Could you check a few things on this model? Use its own coordinates, in mm. Give positions to 0.01 mm unless a question says otherwise; leave off trailing zeros. Loops run counter-clockwise (first coordinate to the right, second up) from the corner with the lowest first, then second, coordinate; pieces in that order, holes last. Notation, with made-up numbers: (27.5, -37.5) - (55.5, -37.5) arc R25 cw to (55.5, -3.5) - close; hole circle Ø1 at (60.5, -20.75). An arc over 180 degrees is marked (long way). Write each question's results on one line, items separated by ' | '. Start each with the question number.
(1) Suppose I cut it at B-B (y = 0.6). Count the separate pieces of the cut face and the enclosed holes in it, and give its area (3 significant figures).
(2) I need wall thicknesses on line 1 (X direction, y = 0.95, z = 8); line 2 (X direction, y = 0.8, z = 3.81); line 3 (X direction, y = 1, z = -2.54). Which ranges of each line are inside material? Lowest first, please.
(3) For pin 1 (5 mm diameter, centred on x = -8, z = 8, fed in from -Y); pin 2 (3 mm diameter, centred on x = 8, z = 8, fed in from +Y), each with a flat end and sliding along its axis, tell me the tip position at first contact or that it passes through.
(4) Suppose I cut it at D-D (z = 1.5). Please give me the cut outline in (x, y), and give its area (3 significant figures).
(5) If we mould it in two halves opening along Z, with no side actions, what happens to faces 1 (the face through (-8.97, 0.79, 6.73)), 2 (the face through (10.737, 0.789, 10.438)), 3 (the face through (11.65, 1, 0))? For each: released by +Z, released by -Z, zero draft, split by the parting line, or undercut.
(6) Suppose I cut it at C-C (x = -9). Please give me the cut outline in (y, z), and give its area (3 significant figures).
(7) Suppose I cut it at A-A (z = -3.81). Please give me the cut outline in (x, y).
from build123d import *

# Parameters (mm, degrees)
SKETCH_1_R      = 1.6
SKETCH_1_R_2    = 0.5
EXTRUDE_1_DEPTH = 1.6


with BuildPart() as part:
    # Эскиз1 → Бобышка-Вытянуть1 (new body)
    with BuildSketch(Plane(origin=(0, 0, 0), x_dir=(1, 0, 0), z_dir=(0, 1, 0))):
        with BuildLine():
            Line((-8.45, 11.4), (8.45, 11.4))
            ThreePointArc((8.45, 11.4), (10.7127417, 10.4627417), (11.65, 8.2))
            Line((11.65, 8.2), (11.65, -8.2))
            ThreePointArc((11.65, -8.2), (10.7127417, -10.4627417), (8.45, -11.4))
            Line((8.45, -11.4), (-8.45, -11.4))
            ThreePointArc((-8.45, -11.4), (-10.7127417, -10.4627417), (-11.65, -8.2))
            Line((-11.65, -8.2), (-11.65, 8.2))
            ThreePointArc((-11.65, 8.2), (-10.7127417, 10.4627417), (-8.45, 11.4))
        make_face()
        with Locations(Location((-8, 8, 0), (0, 0, 270))):
            Circle(SKETCH_1_R, mode=Mode.SUBTRACT)
        with Locations(Location((8, 8, 0), (0, 0, 270))):
            Circle(SKETCH_1_R, mode=Mode.SUBTRACT)
        with Locations(Location((8, -8, 0), (0, 0, 270))):
            Circle(SKETCH_1_R, mode=Mode.SUBTRACT)
        with Locations(Location((-8, -8, 0), (0, 0, 270))):
            Circle(SKETCH_1_R, mode=Mode.SUBTRACT)
        with Locations(Location((-6.65, 0, 0), (0, 0, 270))):
            Circle(SKETCH_1_R_2, mode=Mode.SUBTRACT)
        with Locations(Location((-6.65, -2.54, 0), (0, 0, 270))):
            Circle(SKETCH_1_R_2, mode=Mode.SUBTRACT)
        with Locations(Location((-6.65, 2.54, 0), (0, 0, 270))):
            Circle(SKETCH_1_R_2, mode=Mode.SUBTRACT)
        with Locations(Location((6.65, 3.81, 0), (0, 0, 270))):
            Circle(SKETCH_1_R_2, mode=Mode.SUBTRACT)
        with Locations(Location((6.65, 1.27, 0), (0, 0, 270))):
            Circle(SKETCH_1_R_2, mode=Mode.SUBTRACT)
        with Locations(Location((6.65, -1.27, 0), (0, 0, 270))):
            Circle(SKETCH_1_R_2, mode=Mode.SUBTRACT)
        with Locations(Location((6.65, -3.81, 0), (0, 0, 270))):
            Circle(SKETCH_1_R_2, mode=Mode.SUBTRACT)
    extrude(amount=EXTRUDE_1_DEPTH)


solid = part.part
Output values:
1) separate pieces: 1 | enclosed holes: 11 | area: 485 mm2
2) line 1: -11.65 to -9.6, -6.4 to 6.4, 9.6 to 11.65 | line 2: -11.65 to 6.15, 7.15 to 11.65 | line 3: -11.65 to -7.15, -6.15 to 11.65
3) pin 1: y = 0 | pin 2: through
4) outline: (-11.65, 0) - (6.21, 0) - (6.21, 1.6) - (-11.65, 1.6) - close; (7.09, 0) - (11.65, 0) - (11.65, 1.6) - (7.09, 1.6) - close | area: 35.9 mm2
5) face 1: undercut | face 2: released by +Z | face 3: zero draft
6) outline: (0, -11.35) - (1.6, -11.35) - (1.6, -9.25) - (0, -9.25) - close; (0, -6.75) - (1.6, -6.75) - (1.6, 6.75) - (0, 6.75) - close; (0, 9.25) - (1.6, 9.25) - (1.6, 11.35) - (0, 11.35) - close | area: 28.3 mm2
7) outline: (-11.65, 0) - (6.15, 0) - (6.15, 1.6) - (-11.65, 1.6) - close; (7.15, 0) - (11.65, 0) - (11.65, 1.6) - (7.15, 1.6) - close
